Autodesk Inventor part; units mm, degrees
ref_plane "YZ Plane" through (0, 0, 0) normal (1, 0, 0) x (0, 1, 0)
ref_plane "XZ Plane" through (0, 0, 0) normal (0, 1, 0) x (-1, 0, 0)
ref_plane "XY Plane" through (0, 0, 0) normal (0, 0, 1) x (1, 0, 0)
sketch "Esboço1" plane through (0, 0, 0) normal (0, 1, 0) x (-1, 0, 0)
  line L0 (-21.5, 21.5) -> (-21.5, -21.5)
  line L1 (21.5, -21.5) -> (21.5, 21.5)
  line L2 (21.5, 21.5) -> (-21.5, -21.5) construction
  line L3 (-21.5, 21.5) -> (21.5, -21.5) construction
  line L4 (21.5, -21.5) -> (14.5, -21.5)
  line L5 (14.5, -21.5) -> (0, -18.5)
  line L6 (-21.5, -21.5) -> (-14.5, -21.5)
  line L7 (-14.5, -21.5) -> (0, -18.5)
  line L8 (-21.5, -21.5) -> (-14.5, -21.5)
  line L9 (14.5, -21.5) -> (21.5, -21.5)
  line L10 (21.5, 21.5) -> (14.5, 21.5)
  line L11 (14.5, 21.5) -> (0, 18.5)
  line L12 (-21.5, 21.5) -> (-14.5, 21.5)
  line L13 (-14.5, 21.5) -> (0, 18.5)
  line L14 (20, -20) -> (20, 20)
  line L15 (20, 20) -> (14.6535, 20)
  line L16 (14.6535, 20) -> (0, 16.9682)
  line L17 (0, 16.9682) -> (-14.6535, 20)
  line L18 (-14.6535, 20) -> (-20, 20)
  line L19 (-20, 20) -> (-20, -20)
  line L20 (20, -20) -> (14.6535, -20)
  line L21 (14.6535, -20) -> (0, -16.9682)
  line L22 (0, -16.9682) -> (-14.6535, -20)
  line L23 (-14.6535, -20) -> (-20, -20)
  line L24 (20, 20) -> (20, 21.5)
  line L25 (20, -20) -> (20, -21.5)
  line L26 (-20, -20) -> (-20, -21.5)
  line L27 (-20, 20) -> (-20, 21.5)
  point P0 (0, 0)
  dimension "d0" = 43
  dimension "d1" = 43
  dimension "d2" = 37
  dimension "d3" = 7
  dimension "d4" = 7
extrude "Extrusão1" add sketch "Esboço1" along normal blind 23 contours L12 L27 L19 L26 L6 L0 | L10 L1 L4 L25 L14 L24
extrude "Extrusão2" add sketch "Esboço1" along normal blind 1 contours L12 L13 L11 L10 L24 L15 L16 L17 L18 L27 | L26 L23 L22 L21 L20 L25 L4 L5 L7 L6 | L18 L17 L16 L15 L14 L20 L21 L22 L23 L19
sketch "Esboço2" plane through (-21.5, 0, -21.5) normal (-1, 0, 0) x (0, 0, 1)
  line L0 (0, 0) -> (0, 23)
  line L1 (0, 23) -> (0, 18)
  line L2 (3, 0) -> (0, 0)
  line L3 (0, 0) -> (0, 5)
  line L4 (0, 11.5) -> (43, 11.5)
  line L5 (43, 0) -> (43, 23)
  line L6 (3, 11.5) -> (40, 11.5)
  line L7 (3, 16.5) -> (3, 6.5)
  line L8 (0, 18) -> (3, 16.5)
  line L9 (0, 5) -> (3, 6.5)
  line L10 (0, 18) -> (0, 5)
  line L11 (43, 23) -> (0, 23)
  line L12 (21.5, 23) -> (21.5, 0)
  line L13 (43, 23) -> (43, 18)
  line L14 (43, 0) -> (43, 5)
  line L15 (40, 16.5) -> (40, 6.5)
  line L16 (43, 18) -> (40, 16.5)
  line L17 (43, 5) -> (40, 6.5)
  line L18 (43, 18) -> (43, 5)
  line L19 (43, 0) -> (0, 0)
  line L20 (43, 0) -> (38, 0)
  line L21 (43, 5) -> (43, 0)
  circle A0 centre (38, 3) radius 1
  circle A1 centre (38, 20) radius 1
  circle A2 centre (5, 3) radius 1
  circle A3 centre (5, 20) radius 1
  line L22 (0, 11.5) -> (8, 11.5)
  line L23 (8, 11.5) -> (9, 11.5)
  circle A4 centre (9, 11.5) radius 1
  line L24 (43, 11.5) -> (34, 11.5)
  circle A5 centre (34, 11.5) radius 1
  point P0 (21.5, 11.5)
  dimension "d15" = 5
  dimension "d16" = 5
  dimension "d17" = 37
  dimension "d18" = 10
  dimension "d26" = 2
  dimension "d29" = 17
  dimension "d32" = 33
  dimension "d35" = 8
  dimension "d36" = 1
  dimension "d37" = 2
  dimension "d38" = 3
  dimension "d39" = 5
  dimension "d40" = 9
  dimension "d41" = 2
extrude "Extrusão3" cut sketch "Esboço2" along normal blind 1 and the other way blind 60.75 contours L0 L4 L7 L9 | L0 L8 L7 L4 | L17 L15 L4 L5 | L15 L16 L5 L4
extrude "Extrusão4" cut sketch "Esboço2" against normal blind 3 contours A4 L4 | L4 A4 | A5 L4 | L4 A5 | A0 | A1 | A2 | A3
sketch "Esboço5" plane through (21.5, 0, 21.5) normal (1, 0, 0) x (0, 0, -1)
  line L0 (11.5, 0) -> (31.5, 0)
  line L1 (0, 0) -> (43, 0)
  line L2 (11.5, 0) -> (11.5, 4)
  line L3 (31.5, 0) -> (31.5, 3)
  circle A0 centre (11.5, 4) radius 1
  circle A1 centre (31.5, 4) radius 1
  circle A2 centre (11.5, 19) radius 1
  circle A3 centre (31.5, 19) radius 1
  line L4 (0, 23) -> (43, 23)
  point P0 (21.5, 0)
  dimension "d46" = 3
  dimension "d47" = 2
  dimension "d50" = 20
  dimension "d53" = 15
  dimension "d56" = 4
extrude "Extrusão5" cut sketch "Esboço5" against normal blind 3
fillet "Arredondamento2" radius 0.5 14 edges at (-20, 1, 0) (20, 1, 0) (-20.75, 23, -21.5) (-20.75, 18, -21.5) (-20.75, 5, -21.5) (20.75, 5, -21.5) (20.75, 18, -21.5) (20.75, 23, -21.5) (20.75, 23, 21.5) (20.75, 18, 21.5) (20.75, 5, 21.5) (-20.75, 5, 21.5) (-20.75, 18, 21.5) (-20.75, 23, 21.5)
properties part number "BiaFrame"
Could you check a few things on this model? Use its own coordinates, in mm. A direction names the side the tool comes from. Give positions to 0.01 mm unless a question says otherwise; leave off trailing zeros. Loops run counter-clockwise (first coordinate to the right, second up) from the corner with the lowest first, then second, coordinate; pieces in that order, holes last. Notation, with made-up numbers: M -30,55.25 L -3,55.25 A16 ccw -3,82.25 Z; hole C 59,70.5 d3. An arc over 180 degrees is marked long. Answer as a JSON object with one key per item and string values.
Q1. Suppose I cut it at D-D, the plane z = 0.5. List the corners of the cut face in (x, y) for me, plus the area to 3 significant figures.
Values found:
{"outline": "M -21.5,0 L 21.5,0 L 21.5,23 L 20,23 L 20,1.5 A0.5 cw 19.5,1 L -19.5,1 A0.5 cw -20,1.5 L -20,23 L -21.5,23 Z", "area": "109 mm²"}
Q2. Suppose I cut it at B-B, the plane z = -12.5. List the corners of the cut face in (x, y) for me.
Values found:
{"outline": "M -21.5,0 L 21.5,0 L 21.5,23 L 20,23 L 20,1.5 A0.5 cw 19.5,1 L -19.5,1 A0.5 cw -20,1.5 L -20,10.5 L -21.5,10.5 Z; M -21.5,12.5 L -20,12.5 L -20,23 L -21.5,23 Z"}
Q3. For faces 1 (the flat face through (-20, 12, 0)), 2 (the cylindrical face through (-20.76, 3.3, -15.546)), 3 (the flat face through (20.8, 17.2, -19.9)), which set-ups out of +Z, -Z, +X, -X, +Y, -Y let a thin tool reach every point of the face, with its end or its side?
Values found:
{"face 1": "+Z, -Z, +Y", "face 2": "-X", "face 3": "-Z, +X, -X"}
Q4. If I drill on probe 1 along Z at (x, y) = (21.15, 4); probe 2 along Z at (x, y) = (-20.7, 11.5); probe 3 along X at (y, z) = (14.75, -18), over which ranges is the centre line in solid material (lowest first)? Write a range as [from, to].
Values found:
{"probe 1": "z = [-21.5, -11], [-9, 9], [11, 21.5]", "probe 2": "z = [-18.5, -13.5], [-11.5, 11.5], [13.5, 18.5]", "probe 3": "x = [-21.5, -20], [20, 21.5]"}
Q5. For P1, Ø2.5, axis at y = 4, z = -10, coming from the +X side; P2, Ø1.2, axis at x = -20.5, y = 13.5, coming from the -Z side; P3, Ø12, axis at x = -2.5, y = 3.5, coming from the -Z side, each with a flat end and sliding along its axis, tell me the tip position at first contact or that it passes through.
Values found:
{"P1": "stops at x = 21.5", "P2": "stops at z = -18.5", "P3": "stops at z = -20.15"}
Q6. Suppose I cut it at C-C, the plane y = 11.5. List the corners of the cut face in (x, z) for me.
Values found:
{"outline": "M -21.5,-18.5 L -20,-18.5 L -20,-13.5 L -21.5,-13.5 Z; M -21.5,-11.5 L -20,-11.5 L -20,11.5 L -21.5,11.5 Z; M -21.5,13.5 L -20,13.5 L -20,18.5 L -21.5,18.5 Z; M 20,-18.5 L 21.5,-18.5 L 21.5,18.5 L 20,18.5 Z"}
Q7. Suppose I cut it at A-A, the plane y = 21.75. List the corners of the cut face in (x, z) for me.
Values found:
{"outline": "M -21.5,-21.5 L -20,-21.5 L -20,21.5 L -21.5,21.5 Z; M 20,-21.5 L 21.5,-21.5 L 21.5,21.5 L 20,21.5 Z"}
Q8. If we mould it in two halves opening along Y, with no side actions, what happens to faces 4 (the flat face through (20.8, 17.2, 19.9)), 5 (the flat face through (-21.5, 11, 0)), 6 (the flat face through (-21, 23, 0))? For each: pulls with the +Y half, pulls with the -Y half, needs draft (parallel to the pull), parting line crosses it, or undercut.
Values found:
{"face 4": "undercut", "face 5": "needs draft", "face 6": "pulls with the +Y half"}
